from build123d import *

# Parameters (mm, degrees)
SKETCH1_W                                         = 127
SKETCH1_H                                         = 15.875
SKETCH1_R                                         = 4.7625
BOSS_EXTRUDE1_DEPTH                               = 6.35
CSK_FOR_6_FLAT_HEAD_MACHINE_SCREW_100_D           = 3.7973
CSK_FOR_6_FLAT_HEAD_MACHINE_SCREW_100_CSINK_D     = 7.0866
CSK_FOR_6_FLAT_HEAD_MACHINE_SCREW_100_CSINK_ANGLE = 100
SKETCH5_W                                         = 6.35
SKETCH5_H                                         = 12.7
CUT_EXTRUDE1_DEPTH                                = 103.107229941
SKETCH6_W                                         = 6.35
SKETCH6_H                                         = 1.5875
CUT_EXTRUDE2_DEPTH                                = 103.107229941
TAP_DRILL_FOR_6_32_TAP1_D                         = 2.7051
TAP_DRILL_FOR_6_32_TAP1_DEPTH                     = 6.35
TAP_DRILL_FOR_6_32_TAP1_TIP                       = 0.81269403


with BuildPart() as part:
    # Sketch1 → Boss-Extrude1 (new body)
    with BuildSketch(Plane.XY):
        with Locations((-38.1, 0)):
            Rectangle(SKETCH1_W, SKETCH1_H)
        Polygon((-88.9, 3.476766434), (-66.880479253, 0), (-88.9, -3.476766434), align=None, mode=Mode.SUBTRACT)
        Polygon((-80.757020747, -4.7625), (-58.7375, -1.285733566), (-36.717979253, -4.7625), align=None, mode=Mode.SUBTRACT)
        Polygon((-28.575, -3.476766434), (-50.594520747, 0), (-28.575, 3.476766434), align=None, mode=Mode.SUBTRACT)
        Polygon((-36.717979253, 4.7625), (-58.7375, 1.285733566), (-80.757020747, 4.7625), align=None, mode=Mode.SUBTRACT)
        Circle(SKETCH1_R, mode=Mode.SUBTRACT)
    extrude(amount=BOSS_EXTRUDE1_DEPTH)

    # CSK for #6 Flat Head Machine Screw (100)1 (through all)
    with Locations(Plane(origin=(0, 0, 0), x_dir=(-1, 0, 0), z_dir=(0, 0, -1))):
        with Locations((-22.225, 0), (22.225, 0)):
            CounterSinkHole(CSK_FOR_6_FLAT_HEAD_MACHINE_SCREW_100_D / 2, CSK_FOR_6_FLAT_HEAD_MACHINE_SCREW_100_CSINK_D / 2, counter_sink_angle=CSK_FOR_6_FLAT_HEAD_MACHINE_SCREW_100_CSINK_ANGLE)

    # Sketch5 → Cut-Extrude1 (cut, through all)
    with BuildSketch(Plane(origin=(0, 0, 0), x_dir=(-1, 0, 0), z_dir=(0, 0, -1))):
        with Locations((98.425, 0)):
            Rectangle(SKETCH5_W, SKETCH5_H)
    extrude(amount=-CUT_EXTRUDE1_DEPTH, mode=Mode.SUBTRACT)

    # Sketch6 → Cut-Extrude2 (cut, through all)
    with BuildSketch(Plane(origin=(0, 0, 0), x_dir=(-1, 0, 0), z_dir=(0, 0, -1))):
        with Locations((22.225, 7.14375)):
            Rectangle(SKETCH6_W, SKETCH6_H)
        with Locations((-22.225, 7.14375)):
            Rectangle(SKETCH6_W, SKETCH6_H)
    cut_extrude2 = extrude(amount=-CUT_EXTRUDE2_DEPTH, mode=Mode.SUBTRACT)

    # Mirror3: Cut-Extrude2 across plane
    add(cut_extrude2.mirror(Plane(origin=(0, 3.046697428, 2.281546151), x_dir=(0, -0.5994152204724752, 0.8004382508763147), z_dir=(0, -0.8004382508763147, -0.5994152204724751))), mode=Mode.SUBTRACT)

    # Tap Drill for #6-32 Tap1
    with Locations(Plane.ZY.offset(95.25)):
        with Locations((3.175, 0)):
            Hole(TAP_DRILL_FOR_6_32_TAP1_D / 2, depth=TAP_DRILL_FOR_6_32_TAP1_DEPTH)
            with Locations((0, 0, -(TAP_DRILL_FOR_6_32_TAP1_DEPTH + TAP_DRILL_FOR_6_32_TAP1_TIP / 2))):  # 118° drill point
                Cone(0, TAP_DRILL_FOR_6_32_TAP1_D / 2, TAP_DRILL_FOR_6_32_TAP1_TIP, mode=Mode.SUBTRACT)


solid = part.part
Geometry check sheet. Reference: the model listing, model coordinates, mm. A direction names the side the tool comes from. Coordinates: 2 decimals unless noted, no trailing zeros. Order: outer loops, then holes, each group sorted by start corner. A loop starts at its lowest first (then second) coordinate and runs counter-clockwise, first axis right, second up. Notation, with made-up numbers: (-28.5, 18.25) -> (-11.5, 18.25) arc R13 ccw to (-11.5, 27.25) -> close; hole circle Ø3 at (52, 29). An arc over 180 degrees is marked (long way). Use a Markdown table: item, result. Add a question column.
1. Cross-section at B-B (x = -72). Enter the section's corners in (y, z), and give its area (3 significant figures).
2. Go/stop test with flat-tipped pins: pin 1 Ø0.5 at (y, z) = (7, 3) entering from +X; pin 2 Ø1.5 at (y, z) = (3.5, 1) entering from -X; pin 3 Ø3 at (x, z) = (21, 2) entering from +Y. Record where each tip stops, or that it passes through.
3. Material ranges on L1, parallel to Y at x = -47.5, z = 1.25; L2, parallel to X at y = -7, z = 0.75; L3, parallel to Z at x = -91.5, y = 0, recorded low to high.
4. Mould release check, pull along Y, two halves, no side actions. Record for faces 5 (the face through (-28.575, 0, 3)), 6 (the face through (22, 6.35, 3)), 7 (the face through (-39.431, -1.763, 3.131)), 8 (the face through (25.4, -1, 3)): pulls with the +Y half, pulls with the -Y half, needs draft (parallel to the pull), parting line crosses it, or undercut.
5. Cross-section at A-A (x = 0). Enter the section's corners in (y, z).
6. Set-up check for faces 1 (the face through (19.05, -5, 1)), 2 (the face through (-25.4, -5, 1)), 3 (the face through (-98, -6.35, 3)), 4 (the face through (-92.031, 0.059, 4.526)): record each of +Z, -Z, +X, -X, +Y, -Y from which the full face is reachable in a straight line by a thin tool's end or side.
Filled sheet:
| question | item | result |
|---|---|---|
| 1 | outline | (-7.94, 0) -> (-4.76, 0) -> (-4.76, 6.35) -> (-7.94, 6.35) -> close; (-3.38, 0) -> (-0.81, 0) -> (-0.81, 6.35) -> (-3.38, 6.35) -> close; (0.81, 0) -> (3.38, 0) -> (3.38, 6.35) -> (0.81, 6.35) -> close; (4.76, 0) -> (7.94, 0) -> (7.94, 6.35) -> (4.76, 6.35) -> close |
| 1 | area | 73.0 mm2 |
| 2 | pin 1 | x = 19.05 |
| 2 | pin 2 | x = -95.25 |
| 2 | pin 3 | y = 6.35 |
| 3 | L1 | -7.94 to -4.76, -3.06 to -0.49, 0.49 to 3.06, 4.76 to 7.94 |
| 3 | L2 | -101.6 to -25.4, -19.05 to 19.05 |
| 3 | L3 | 0 to 1.82, 4.53 to 6.35 |
| 4 | face 5 | undercut |
| 4 | face 6 | pulls with the +Y half |
| 4 | face 7 | undercut |
| 4 | face 8 | needs draft |
| 5 | outline | (-7.94, 0) -> (-4.76, 0) -> (-4.76, 6.35) -> (-7.94, 6.35) -> close; (4.76, 0) -> (7.94, 0) -> (7.94, 6.35) -> (4.76, 6.35) -> close |
| 6 | face 1 | +X |
| 6 | face 2 | none |
| 6 | face 3 | +Z, -Z, -X |
| 6 | face 4 | -X |
